The listing builds one solid part. Answer for the finished solid, in the listing's coordinates (mm). A direction names the side the tool comes from. Coordinates: 2 decimals unless noted, no trailing zeros. Loops run counter-clockwise (first coordinate to the right, second up) from the corner with the lowest first, then second, coordinate; pieces in that order, holes last. Notation, with made-up numbers: (18, 68.25) - (48, 68.25) arc R23 cw to (48, 77.25) - close; hole circle Ø5 at (10, -4). An arc over 180 degrees is marked (long way). Put each result on its own line as item: value.
```python
from build123d import *

# Parameters (mm, degrees)
SKETCH1_W            = 12.7
SKETCH1_H            = 18.796
BOSS_EXTRUDE1_DEPTH  = 6.35
SKETCH2_R            = 2.5527
CUT_EXTRUDE1_DEPTH   = 6.35
SKETCH3_W            = 66.04
SKETCH3_H            = 6.35
BOSS_EXTRUDE2_DEPTH  = 5.08
SKETCH4_W            = 40.64
SKETCH4_H            = 1.524
BOSS_EXTRUDE5_DEPTH  = 3.81
SKETCH9_W            = 40.64
SKETCH9_H            = 30.988
BOSS_EXTRUDE6_DEPTH  = 3.81
SKETCH10_W           = 53.34
SKETCH10_H           = 6.35
CUT_EXTRUDE3_DEPTH   = 1.27
SKETCH11_W           = 12.7
SKETCH11_H           = 19.05
BOSS_EXTRUDE7_DEPTH  = 1.27
SKETCH16_R           = 2.5527
CUT_EXTRUDE5_DEPTH   = 1.27
SKETCH17_W           = 12.7
SKETCH17_H           = 6.35
BOSS_EXTRUDE8_DEPTH  = 23.876
SKETCH20_R           = 2.5527
CUT_EXTRUDE6_DEPTH   = 6.35
SKETCH21_W           = 12.7
SKETCH21_H           = 19.05
BOSS_EXTRUDE9_DEPTH  = 1.27
SKETCH22_R           = 2.5527
CUT_EXTRUDE7_DEPTH   = 1.27
SKETCH23_W           = 40.64
SKETCH23_H           = 23.876
BOSS_EXTRUDE10_DEPTH = 1.27
SKETCH24_W           = 40.64
SKETCH24_H           = 13.97
BOSS_EXTRUDE11_DEPTH = 1.27
SKETCH25_R           = 2.5527
CUT_EXTRUDE8_DEPTH   = 1.27
FILLET4_R            = 6.35
FILLET5_R            = 0.254


with BuildPart() as part:
    # Sketch1 → Boss-Extrude1 (new body)
    with BuildSketch(Plane(origin=(0, 0, 0), x_dir=(1, 0, 0), z_dir=(0, 1, 0))):
        with Locations((6.35, 9.398)):
            Rectangle(SKETCH1_W, SKETCH1_H)
    extrude(amount=BOSS_EXTRUDE1_DEPTH)

    # Sketch2 → Cut-Extrude1 (cut)
    with BuildSketch(Plane(origin=(0, 6.35, 0), x_dir=(1, 0, 0), z_dir=(0, 1, 0))):
        with Locations(Location((8.552562419, 14.75, 0), (0, 0, 270))):
            Circle(SKETCH2_R)
        with Locations(Location((8.552562419, 5.25, 0), (0, 0, 270))):
            Circle(SKETCH2_R)
    extrude(amount=-CUT_EXTRUDE1_DEPTH, mode=Mode.SUBTRACT)

    # Sketch3 → Boss-Extrude2 (add)
    with BuildSketch(Plane(origin=(0, 0, -18.796), x_dir=(-1, 0, 0), z_dir=(0, 0, -1))):
        with Locations((-33.02, 3.175)):
            Rectangle(SKETCH3_W, SKETCH3_H)
    extrude(amount=BOSS_EXTRUDE2_DEPTH)

    # Sketch4 → Boss-Extrude5 (add)
    with BuildSketch(Plane(origin=(0, 0, -23.876), x_dir=(-1, 0, 0), z_dir=(0, 0, -1))):
        with Locations((-33.02, 7.112)):
            Rectangle(SKETCH4_W, SKETCH4_H)
    extrude(amount=-BOSS_EXTRUDE5_DEPTH)

    # Sketch9 → Boss-Extrude6 (add)
    with BuildSketch(Plane(origin=(0, 0, -23.876), x_dir=(-1, 0, 0), z_dir=(0, 0, -1))):
        with Locations((-33.02, -15.494)):
            Rectangle(SKETCH9_W, SKETCH9_H)
    extrude(amount=-BOSS_EXTRUDE6_DEPTH)

    # Sketch10 → Cut-Extrude3 (cut)
    with BuildSketch(Plane.XY.offset(-18.796)):
        with Locations((39.37, 3.175)):
            Rectangle(SKETCH10_W, SKETCH10_H)
    extrude(amount=-CUT_EXTRUDE3_DEPTH, mode=Mode.SUBTRACT)

    # Sketch11 → Boss-Extrude7 (add)
    with BuildSketch(Plane.XY):
        with Locations((6.35, 9.525)):
            Rectangle(SKETCH11_W, SKETCH11_H)
    extrude(amount=-BOSS_EXTRUDE7_DEPTH)

    # Sketch16 → Cut-Extrude5 (cut)
    with BuildSketch(Plane(origin=(0, 0, -1.27), x_dir=(-1, 0, 0), z_dir=(0, 0, -1))):
        with Locations((-6.35, 12.7)):
            Circle(SKETCH16_R)
    extrude(amount=-CUT_EXTRUDE5_DEPTH, mode=Mode.SUBTRACT)

    # Sketch17 → Boss-Extrude8 (add)
    with BuildSketch(Plane(origin=(0, 0, -23.876), x_dir=(-1, 0, 0), z_dir=(0, 0, -1))):
        with Locations((-59.69, 3.175)):
            Rectangle(SKETCH17_W, SKETCH17_H)
    extrude(amount=-BOSS_EXTRUDE8_DEPTH)

    # Sketch20 → Cut-Extrude6 (cut)
    with BuildSketch(Plane(origin=(0, 6.35, 0), x_dir=(1, 0, 0), z_dir=(0, 1, 0))):
        with Locations(Location((57.247437581, 14.75, 0), (0, 0, 270))):
            Circle(SKETCH20_R)
        with Locations(Location((57.247437581, 5.25, 0), (0, 0, 270))):
            Circle(SKETCH20_R)
    extrude(amount=-CUT_EXTRUDE6_DEPTH, mode=Mode.SUBTRACT)

    # Sketch21 → Boss-Extrude9 (add)
    with BuildSketch(Plane.XY):
        with Locations((59.69, 9.525)):
            Rectangle(SKETCH21_W, SKETCH21_H)
    extrude(amount=-BOSS_EXTRUDE9_DEPTH)

    # Sketch22 → Cut-Extrude7 (cut)
    with BuildSketch(Plane(origin=(0, 0, -1.27), x_dir=(-1, 0, 0), z_dir=(0, 0, -1))):
        with Locations((-59.69, 12.7)):
            Circle(SKETCH22_R)
    extrude(amount=-CUT_EXTRUDE7_DEPTH, mode=Mode.SUBTRACT)

    # Sketch23 → Boss-Extrude10 (add)
    with BuildSketch(Plane.XZ.offset(30.988)):
        with Locations((33.02, -11.938)):
            Rectangle(SKETCH23_W, SKETCH23_H)
    extrude(amount=BOSS_EXTRUDE10_DEPTH)

    # Sketch24 → Boss-Extrude11 (add)
    with BuildSketch(Plane.XY):
        with Locations((33.02, -37.973)):
            Rectangle(SKETCH24_W, SKETCH24_H)
    extrude(amount=-BOSS_EXTRUDE11_DEPTH)

    # Sketch25 → Cut-Extrude8 (cut)
    with BuildSketch(Plane(origin=(0, 0, -1.27), x_dir=(-1, 0, 0), z_dir=(0, 0, -1))):
        with Locations((-46.99, -38.608)):
            Circle(SKETCH25_R)
        with Locations((-19.05, -38.608)):
            Circle(SKETCH25_R)
    extrude(amount=-CUT_EXTRUDE8_DEPTH, mode=Mode.SUBTRACT)

    # Fillet4
    fillet4_edges = [part.edges().sort_by_distance(p)[0] for p in [
        (0, 3.175, -23.876),
        (66.04, 3.175, -23.876),
    ]]
    fillet(fillet4_edges, radius=FILLET4_R)

    # Fillet5
    fillet5_edges = [part.edges().sort_by_distance(p)[0] for p in [
        (59.69, 6.35, -1.27),
        (33.02, -32.258, -23.876),
        (33.02, -32.258, -1.27),
        (53.34, 7.112, -23.876),
        (12.7, 7.112, -23.876),
        (33.02, 7.874, -23.876),
        (12.7, -16.129, -23.876),
        (53.34, -16.129, -23.876),
        (6.35, 6.35, -1.27),
    ]]
    fillet(fillet5_edges, radius=FILLET5_R)


solid = part.part
```
1) Each of these flat-tipped pins is pushed along its axis until it touches: pin 1 (6 mm diameter, centred on x = 56.5, y = 12, fed in from -Z); pin 2 (6.5 mm diameter, centred on x = 4.5, z = -11.5, fed in from -Y); pin 3 (3 mm diameter, centred on x = 57.25, z = -5.25, fed in from +Y); pin 4 (3 mm diameter, centred on x = 56.5, z = -17, fed in from +Y). Where does it stop, or does it pass through?
Found:
pin 1: stops at z = -1.27
pin 2: stops at y = 0
pin 3: passes through
pin 4: stops at y = 6.35
2) Straight lines are drawn through the part: L1, parallel to X at y = 5.25, z = -5.25; L2, parallel to Y at x = 19.05, z = -0.5; L3, parallel to Z at x = 52, y = -4. For each, find the intervals that lie inside material, in ascending order. Write a range as [from, to].
Found:
L1: x = [0, 6], [11.11, 12.7], [53.34, 54.69], [59.8, 66.04]
L2: y = [-44.96, -41.16], [-36.06, -30.99]
L3: z = [-23.88, -20.07]
3) The part is cut by section A-A (z = -14.75). Give the vertices of the cut face in (x, y).
Found:
outline: (0, 0) - (6, 0) - (6, 6.35) - (0, 6.35) - close; (11.11, 0) - (12.7, 0) - (12.7, 6.35) - (11.11, 6.35) - close; (12.7, -32.26) - (53.34, -32.26) - (53.34, -30.99) - (12.7, -30.99) - close; (53.34, 0) - (54.69, 0) - (54.69, 6.35) - (53.34, 6.35) - close; (59.8, 0) - (66.04, 0) - (66.04, 6.35) - (59.8, 6.35) - close
4) For a pull along X with two mould halves and no side action, classify faces 1 (the face through (7, 0, -12)), 2 (the face through (64.13, 3.219, -22.065)), 3 (the face through (59.78, 3.22, -15.08)), 4 (the face through (57.255, 13.467, -0.644)) as pulls with the +X half, pulls with the -X half, needs draft (parallel to the pull), parting line crosses it, or undercut.
Found:
face 1: needs draft
face 2: pulls with the +X half
face 3: undercut
face 4: undercut
5) The part is cut by section D-D (x = 10). Give the vertices of the cut face in (y, z), and give its area (3 significant figures).
Found:
outline: (0, -23.88) - (6.35, -23.88) - (6.35, -16.85) - (0, -16.85) - close; (0, -12.65) - (6.35, -12.65) - (6.35, -7.35) - (0, -7.35) - close; (0, -3.15) - (6.35, -3.15) - (6.35, -1.52) arc R0.25 cw to (6.6, -1.27) - (19.05, -1.27) - (19.05, 0) - (0, 0) - close
area: 114 mm^2
6) The part is cut by section C-C (y = 12.7). Give the vertices of the cut face in (x, z), and give its area (3 significant figures).
Found:
outline: (0, -1.27) - (3.8, -1.27) - (3.8, 0) - (0, 0) - close; (8.9, -1.27) - (12.7, -1.27) - (12.7, 0) - (8.9, 0) - close; (53.34, -1.27) - (57.14, -1.27) - (57.14, 0) - (53.34, 0) - close; (62.24, -1.27) - (66.04, -1.27) - (66.04, 0) - (62.24, 0) - close
area: 19.3 mm^2
7) The part is cut by section B-B (x = 46.99). Give the vertices of the cut face in (y, z), and give its area (3 significant figures).
Found:
outline: (-44.96, -1.27) - (-41.16, -1.27) - (-41.16, 0) - (-44.96, 0) - close; (-36.06, -1.27) - (-32.51, -1.27) arc R0.25 cw to (-32.26, -1.52) - (-32.26, -23.62) arc R0.25 ccw to (-32, -23.88) - (7.62, -23.88) arc R0.25 ccw to (7.87, -23.62) - (7.87, -20.07) - (-30.99, -20.07) - (-30.99, 0) - (-36.06, 0) - close
area: 188 mm^2
8) For faces 5 (the face through (12.7, 7, -22)), 6 (the face through (33, -11, -20.066)), 7 (the face through (33, -32.258, -12)), 8 (the face through (33, -30.988, -10)), 9 (the face through (60, 10, -1.27)), determine the directions among +Z, -Z, +X, -X, +Y, -Y from which every point of the face is accessible in a straight line to the end or side of a thin tool.
Found:
face 5: -Z, -X, +Y
face 6: +Z, +Y
face 7: -Z, +X, -X, -Y
face 8: +Z, +X, -X, +Y
face 9: -Z, +X, -X, +Y
